from build123d import *

# Parameters (mm, degrees)
BLANKSKE_W        = 50
BLANKSKE_H        = 11
BLANK_DEPTH       = 6
TOOTHCUTSIM_DEPTH = 52.546095875
TEETHCUTS_COUNT   = 17
TEETHCUTS_PITCH   = 3.14159265


with BuildPart() as part:
    # BlankSke → Blank (new body)
    with BuildSketch(Plane.XY):
        with Locations((25, 5.5)):
            Rectangle(BLANKSKE_W, BLANKSKE_H)
    extrude(amount=-BLANK_DEPTH)

    # TooCutSkeSim → ToothCutSim (cut, through all)
    with BuildSketch(Plane.XY):
        Polygon((0.44443537, 8.75), (-0.44443537, 8.75), (-1.272613241, 11.0254), (1.272613241, 11.0254), align=None)
    toothcutsim = extrude(amount=-TOOTHCUTSIM_DEPTH, mode=Mode.SUBTRACT)

    # TeethCuts: ToothCutSim ×17
    with Locations(*[(i * TEETHCUTS_PITCH, 0, 0) for i in range(1, TEETHCUTS_COUNT)]):
        add(toothcutsim, mode=Mode.SUBTRACT)


solid = part.part
Model file for the job. Use its own axes, mm. Round coordinates to 2 decimals unless told otherwise and drop trailing zeros. Answer as CSV lines item,"result". Start each with the question number.
1) Slice it at A-A (y = 10). State how many separate pieces and enclosed holes the cut face has, plus the area to 3 significant figures.
2) Mould opens along X. For faces 1 (the face through (25, 4, -6)), 2 (the face through (2.293, 9.859, -2.958)), 3 (the face through (50, 4, -3)) say: +X half, -X half, draft (parallel to the pull), parting line (faces both ways), or undercut.
3) Probe line 1 along Y through (x, z) = (25, -5.65). List the from-to ranges inside material, lowest first.
Filled in:
1,separate pieces,"16"
1,enclosed holes,"0"
1,area,"129 mm2"
2,face 1,"draft"
2,face 2,"undercut"
2,face 3,"+X half"
3,line 1,"y = 0 to 8.75"
